```python
from build123d import *

# Parameters (mm, degrees)
BOSS_EXTRUDE1_DEPTH       = 22.5
M4X0_7_TAPPED_HOLE2_D     = 3.3
BOSS_EXTRUDE3_DEPTH       = 6.3625
M4X0_7_TAPPED_HOLE1_D     = 3.3
M4X0_7_TAPPED_HOLE1_DEPTH = 10
M4X0_7_TAPPED_HOLE1_TIP   = 0.991420021
CUT_EXTRUDE2_DEPTH        = 85
SKETCH2_R                 = 3
CUT_EXTRUDE1_DEPTH        = 50
CUT_EXTRUDE3_START        = -10
CUT_EXTRUDE3_DEPTH        = 4


with BuildPart() as part:
    # Sketch1 → Boss-Extrude1 (new body, symmetric)
    with BuildSketch(Plane.XY):
        with BuildLine():
            Line((-15, 7.5), (-15, 9.5))
            Line((-15, 9.5), (15, 9.5))
            Line((15, 9.5), (15, 7.5))
            ThreePointArc((15, 7.5), (7.5, 0), (15, -7.5))
            Line((15, -7.5), (15, -10))
            Line((15, -10), (-15, -10))
            Line((-15, -10), (-15, -7.5))
            ThreePointArc((-15, -7.5), (-7.5, 0), (-15, 7.5))
        make_face()
    extrude(amount=BOSS_EXTRUDE1_DEPTH, both=True)

    # M4x0.7 Tapped Hole2 (through all)
    with Locations(Plane(origin=(0, -10, 0), x_dir=(-1, 0, 0), z_dir=(0, -1, 0))):
        with Locations((0, -17.5), (0, 17.5)):
            Hole(M4X0_7_TAPPED_HOLE2_D / 2)

    # Sketch7 → Boss-Extrude3 (add, symmetric)
    with BuildSketch(Plane.XY):
        Polygon((-15, -7.5), (-24, -7.5), (-24, -42.5), (-9, -42.5), (-9, -27.5), (8.5, -10), (-15, -10), align=None)
    extrude(amount=BOSS_EXTRUDE3_DEPTH, both=True)

    # M4x0.7 Tapped Hole1
    with Locations(Plane(origin=(-24, 0, 0), x_dir=(0, 0, -1), z_dir=(-1, 0, 0))):
        with Locations((0, 37.5), (0, 22.5)):
            Hole(M4X0_7_TAPPED_HOLE1_D / 2, depth=M4X0_7_TAPPED_HOLE1_DEPTH)
            with Locations((0, 0, -(M4X0_7_TAPPED_HOLE1_DEPTH + M4X0_7_TAPPED_HOLE1_TIP / 2))):  # 118° drill point
                Cone(0, M4X0_7_TAPPED_HOLE1_D / 2, M4X0_7_TAPPED_HOLE1_TIP, mode=Mode.SUBTRACT)

    # Sketch10 → Cut-Extrude2 (cut)
    with BuildSketch(Plane(origin=(0, 0, -6.3625), x_dir=(-1, 0, 0), z_dir=(0, 0, -1))):
        Polygon((15, -10), (24, -19), (24, -7.5), (15, -7.5), align=None)
    extrude(amount=-CUT_EXTRUDE2_DEPTH, mode=Mode.SUBTRACT)

    # Sketch2 → Cut-Extrude1 (cut)
    with BuildSketch(Plane(origin=(0, 9.5, 0), x_dir=(1, 0, 0), z_dir=(0, 1, 0))):
        Circle(SKETCH2_R)
    extrude(amount=-CUT_EXTRUDE1_DEPTH, mode=Mode.SUBTRACT)

    # Sketch11 → Cut-Extrude3 (cut)
    with BuildSketch(Plane(origin=(0, 0, -22.5), x_dir=(-1, 0, 0), z_dir=(0, 0, -1)).offset(CUT_EXTRUDE3_START)):
        with BuildLine():
            Line((-5, 9.5), (-5, 0))
            ThreePointArc((-5, 0), (-7.928932188, -7.071067812), (-15, -10))
            Line((-15, -10), (-3.5, -10))
            Line((-3.5, -10), (-3.5, 9.5))
            Line((-3.5, 9.5), (-5, 9.5))
        make_face()
        with BuildLine():
            Line((3.5, 9.5), (5, 9.5))
            Line((5, 9.5), (5, 0))
            ThreePointArc((5, 0), (7.928932188, -7.071067812), (15, -10))
            Line((15, -10), (3.5, -10))
            Line((3.5, -10), (3.5, 9.5))
        make_face()
    cut_extrude3 = extrude(amount=-CUT_EXTRUDE3_DEPTH, mode=Mode.SUBTRACT)

    # Mirror1: Cut-Extrude3 across plane
    add(cut_extrude3.mirror(Plane.XY), mode=Mode.SUBTRACT)


solid = part.part
```
Read the model definition and answer for the solid it produces. Units are mm, in the model's axes. A direction names the side the tool comes from. Round coordinates to 2 decimals unless told otherwise and drop trailing zeros. Write each loop counter-clockwise with the first axis right and the second up, starting at its lowest first coordinate (ties: lowest second). Pieces come first, ordered by that corner, then holes. Notation, with made-up numbers: (8.25, 36.5) - (34.25, 36.5) arc R18 ccw to (34.25, 63.5) - close; hole circle Ø10 at (25, 74). An arc over 180 degrees is marked (long way). Use CSV: the item, a comma, the result in double quotes.
Q1. Find section A-A, the plane z = 17.5. Write down the section's boundary in (x, y).
Values:
outline,"(-15, -10) - (-1.65, -10) - (-1.65, 9.5) - (-15, 9.5) - (-15, 7.5) arc R7.5 cw to (-15, -7.5) - close; (1.65, -10) - (15, -10) - (15, -7.5) arc R7.5 cw to (15, 7.5) - (15, 9.5) - (1.65, 9.5) - close"
Q2. Straight lines are drawn through the part: line 1 along Z through (x, y) = (0, -5); line 2 along Z through (x, y) = (-18.25, -22.5); line 3 along X through (y, z) = (-26, -2.5). For each, find the intervals that lie inside material, in ascending order.
Values:
line 1,"z = -22.5 to -19.15, -15.85 to -3, 3 to 15.85, 19.15 to 22.5"
line 2,"z = -6.36 to -1.65, 1.65 to 6.36"
line 3,"x = -24 to -7.5"
Q3. Find section D-D, the plane y = -14. Write down the section's boundary in (x, z).
Values:
outline,"(-19, -6.36) - (4.5, -6.36) - (4.5, 6.36) - (-19, 6.36) - close; hole circle Ø6 at (0, 0)"
Q4. Each of these flat-tipped pins is pushed along its axis until it touches: pin 1 Ø6 at (x, y) = (-2.5, -23.5) entering from -Z; pin 2 Ø6.5 at (y, z) = (-35, 0.5) entering from +X; pin 3 Ø12 at (x, z) = (7, 2) entering from -Y; pin 4 Ø2 at (x, z) = (0, -17.5) entering from +Y. Where does it stop, or does it pass through?
Values:
pin 1,"stops at z = -6.36"
pin 2,"stops at x = -9"
pin 3,"stops at y = -17.45"
pin 4,"passes through"
Q5. Determine the mould class of faces 1 (the flat face through (-24, -31, 0)), 2 (the cylindrical face through (-7.85, -6.99, 10.53)), 3 (the conical face through (-13.2, -22.2, -0.1)), 4 (the cylindrical face through (7.5, 0.16, 0.32)) for opening direction Y: +Y half, -Y half, draft (parallel to the pull), parting line (faces both ways), or undercut.
Values:
face 1,"draft"
face 2,"-Y half"
face 3,"undercut"
face 4,"undercut"
Q6. Find section C-C, the plane x = 13.5. Write down the section's boundary in (y, z), then the cut area to 3 significant figures.
Values:
outline,"(-10, -22.5) - (-7.35, -22.5) - (-7.35, 22.5) - (-10, 22.5) - (-10, 12.5) - (-9.89, 12.5) - (-9.89, 8.5) - (-10, 8.5) - (-10, -8.5) - (-9.89, -8.5) - (-9.89, -12.5) - (-10, -12.5) - close; (7.35, -22.5) - (9.5, -22.5) - (9.5, 22.5) - (7.35, 22.5) - close"
area,"215 mm²"
Q7. A tool of negligible diameter and unlimited length cuts with its end or side. For faces 5 (the cylindrical face through (7.85, -6.99, 10.53)), 6 (the conical face through (-13.2, -37.2, -0.1)), 7 (the flat face through (-15, 8, 0)), 8 (the flat face through (-9, -35, 0)), 9 (the flat face through (-3.5, 0, -11)), from which of +Z, -Z, +X, -X, +Y, -Y can it reach the whole face along a straight path? Write none if from no direction.
Values:
face 5,"-Y"
face 6,"-X"
face 7,"+Z, -Z, -X, +Y"
face 8,"+Z, -Z, +X, -Y"
face 9,"+Y, -Y"
Q8. Find section B-B, the plane x = 0. Write down the section's boundary in (y, z).
Values:
outline,"(-18.5, -6.36) - (-10, -6.36) - (-10, -15.85) - (9.5, -15.85) - (9.5, -3) - (-18.5, -3) - close; (-18.5, 3) - (9.5, 3) - (9.5, 15.85) - (-10, 15.85) - (-10, 6.36) - (-18.5, 6.36) - close; (-10, -22.5) - (9.5, -22.5) - (9.5, -19.15) - (-10, -19.15) - close; (-10, 19.15) - (9.5, 19.15) - (9.5, 22.5) - (-10, 22.5) - close"
